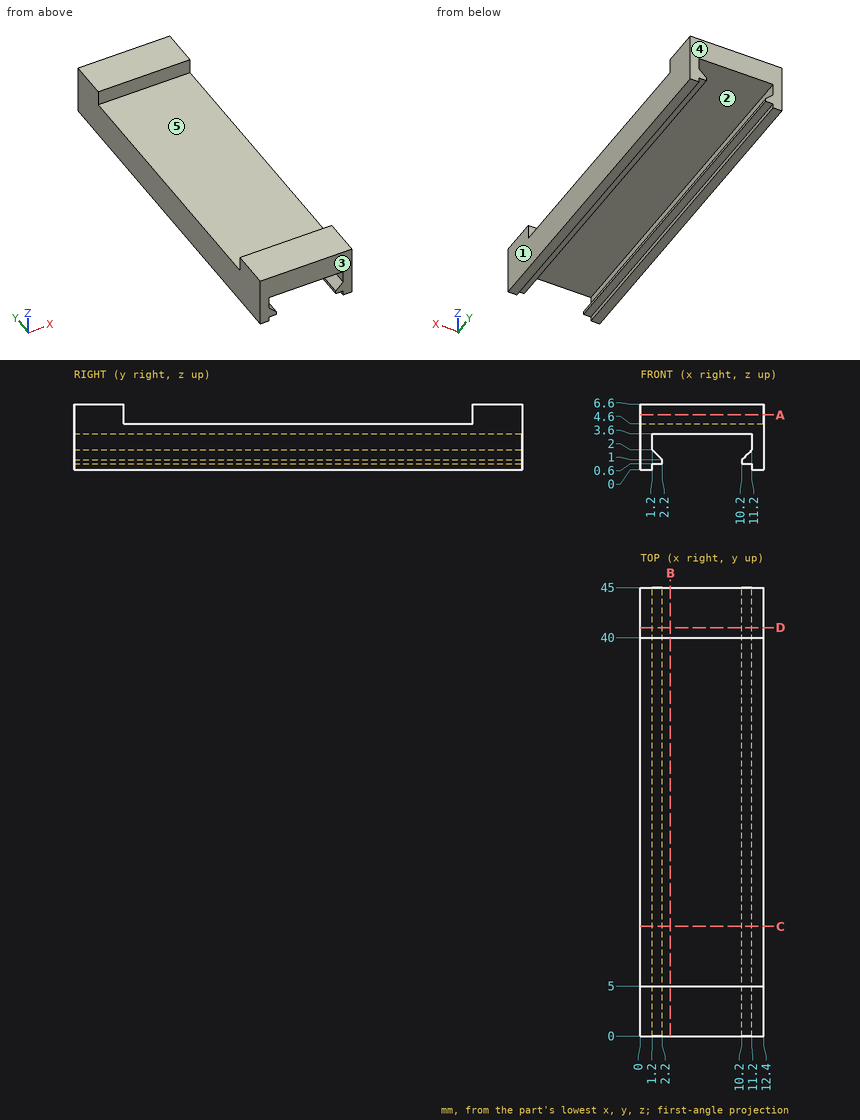
Study the drawing (mm; zero at the part's minimum x, y, z) and answer. A direction names the side the tool comes from. Give positions to 0.01 mm unless a question says otherwise; leave off trailing zeros. Order: outer loops, then holes, each group sorted by start corner. A loop starts at its lowest first (then second) coordinate and runs counter-clockwise, first axis right, second up.
1) Find section B-B on x = 3. Write down the section's boundary in (y, z).
Reported:
outline: (0, 3.6) - (45, 3.6) - (45, 6.6) - (40, 6.6) - (40, 4.6) - (5, 4.6) - (5, 6.6) - (0, 6.6) - close
2) Find section A-A on z = 5.5. Write down the section's boundary in (x, y).
Reported:
outline: (0, 0) - (12.4, 0) - (12.4, 5) - (0, 5) - close; (0, 40) - (12.4, 40) - (12.4, 45) - (0, 45) - close
3) Find section D-D on y = 41. Write down the section's boundary in (x, z), then the cut area to 3 significant figures.
Reported:
outline: (0, 0) - (1.2, 0) - (1.2, 0.6) - (2.2, 0.6) - (2.2, 1) - (1.2, 2) - (1.2, 3.6) - (11.2, 3.6) - (11.2, 2) - (10.2, 1) - (10.2, 0.6) - (11.2, 0.6) - (11.2, 0) - (12.4, 0) - (12.4, 6.6) - (0, 6.6) - close
area: 47.6 mm2
4) Determine the mould class of the marked faces 1, 2 and 3 for opening direction X: pulls with the +X half, pulls with the -X half, needs draft (parallel to the pull), parting line crosses it, or undercut.
Reported:
face 1: pulls with the +X half
face 2: undercut
face 3: needs draft
5) For the marked faces 4 and 5, determine the directions among +Z, -Z, +X, -X, +Y, -Y from which every point of the face is accessible in a straight line to the end or side of a thin tool.
Reported:
face 4: +Z, -Z, +X, -X, +Y
face 5: +Z, +X, -X
6) Consider line 1 along X through (y, z) = (39.5, 2.75); line 2 along Y through (x, z) = (5.75, 5.75); line 3 along Z through (x, y) = (8.5, 24.5). Determine where each line is inside the solid, lowest interval first.
Reported:
line 1: x = 0 to 1.2, 11.2 to 12.4
line 2: y = 0 to 5, 40 to 45
line 3: z = 3.6 to 4.6
7) Find section C-C on y = 11. Write down the section's boundary in (x, z), then the cut area to 3 significant figures.
Reported:
outline: (0, 0) - (1.2, 0) - (1.2, 0.6) - (2.2, 0.6) - (2.2, 1) - (1.2, 2) - (1.2, 3.6) - (11.2, 3.6) - (11.2, 2) - (10.2, 1) - (10.2, 0.6) - (11.2, 0.6) - (11.2, 0) - (12.4, 0) - (12.4, 4.6) - (0, 4.6) - close
area: 22.8 mm2
8) Given P1, Ø6, axis at x = 3.5, y = 22, coming from the +Z side; P2, Ø3, axis at x = 4.5, y = 18, coming from the -Z side; P3, Ø0.8, axis at x = 10.5, y = 19, coming from the -Z side, each flat-ended and moving along its own axis, determine where each tip first touches the part or whether it passes through.
Reported:
P1: stops at z = 4.6
P2: stops at z = 3.6
P3: stops at z = 0.6
